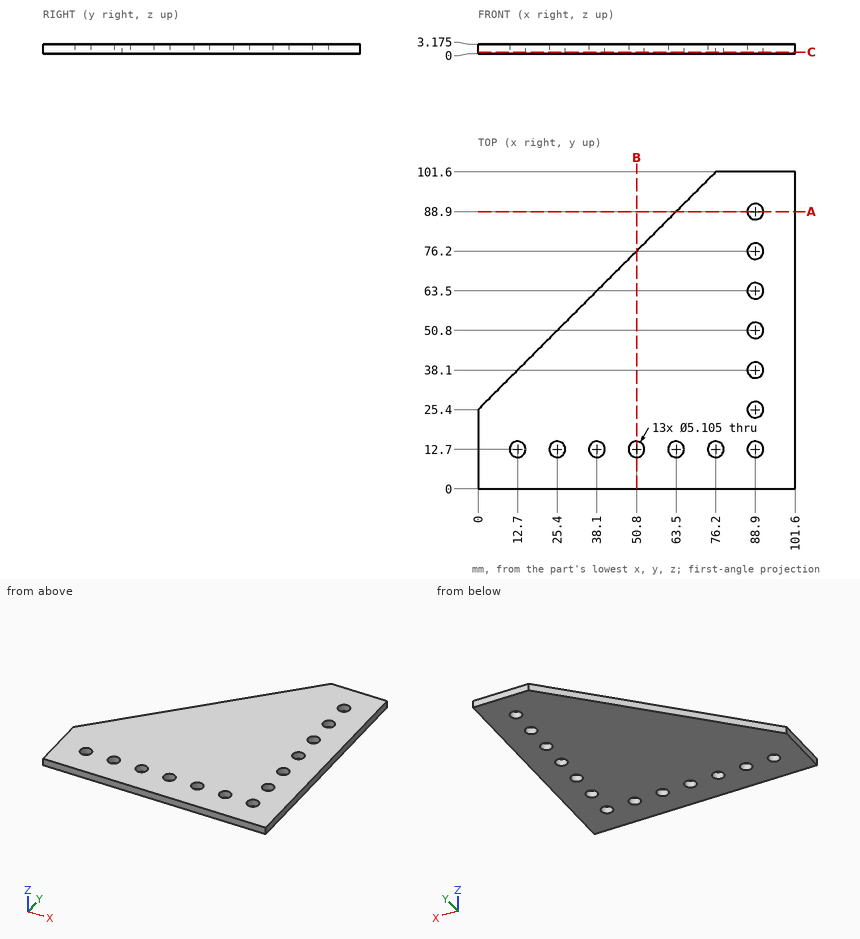
Check sheet for the drawn part. Datum: minimum x, y, z corner. Units: mm. Coordinates: 2 decimals unless noted, no trailing zeros. Write each loop counter-clockwise with the first axis right and the second up, starting at its lowest first coordinate (ties: lowest second). Pieces come first, ordered by that corner, then holes. Notation, with made-up numbers: M 66,55.5 L 77,55.5 A12 ccw 77,71.5 Z; hole C 89,65 d4. An arc over 180 degrees is marked long. Use a Markdown table: item, result.
Q1. Sectioned sample at B-B, the plane x = 50.8. Record the boundary of the cut face in (y, z) (1 decimal).
Reply:
| item | result |
|---|---|
| outline | M 0,0 L 10.1,0 L 10.1,3.2 L 0,3.2 Z; M 15.3,0 L 76.2,0 L 76.2,3.2 L 15.3,3.2 Z |
Q2. Sectioned sample at A-A, the plane y = 88.9. Record the boundary of the cut face in (x, z) (1 decimal), plus the area to 3 significant figures.
Reply:
| item | result |
|---|---|
| outline | M 63.5,0 L 86.3,0 L 86.3,3.2 L 63.5,3.2 Z; M 91.5,0 L 101.6,0 L 101.6,3.2 L 91.5,3.2 Z |
| area | 105 mm² |
Q3. Go/stop test with flat-tipped pins: P1, Ø6.5, axis at x = 63.5, y = 12.7, coming from the -Z side; P2, Ø3, axis at x = 38.1, y = 12.7, coming from the +Z side. Record where each tip stops, or that it passes through.
Reply:
| item | result |
|---|---|
| P1 | stops at z = 0 |
| P2 | passes through |
Q4. Sectioned sample at C-C, the plane z = 0.6. Count the separate pieces of the cut face and the enclosed holes in it, plus the area to 3 significant figures.
Reply:
| item | result |
|---|---|
| separate pieces | 1 |
| enclosed holes | 13 |
| area | 7,150 mm² |
Q5. Thickness scan on line 1 (X direction, y = 27, z = 1.3); line 2 (Y direction, x = 40, z = 2.2) (1 decimal); line 3 (Y direction, x = 64, z = 1.75) (1 decimal). Record the ranges inside material, lowest first.
Reply:
| item | result |
|---|---|
| line 1 | x = 1.6 to 86.91, 90.89 to 101.6 |
| line 2 | y = 0 to 11, 14.4 to 65.4 |
| line 3 | y = 0 to 10.2, 15.2 to 89.4 |
